Here's how the part is built. I have some questions about the finished solid (model axes, mm). Face numbers are marked on the shaded views. A direction names the side the tool comes from. Give positions to 0.01 mm unless a question says otherwise; leave off trailing zeros. Write each loop counter-clockwise with the first axis right and the second up, starting at its lowest first coordinate (ties: lowest second). Pieces come first, ordered by that corner, then holes. Notation, with made-up numbers: (6, 82) -> (35, 82) arc R17 ccw to (35, 97) -> close; hole circle Ø4 at (-7.5, -19). An arc over 180 degrees is marked (long way). Use one line per item in the form item = value.
```python
from build123d import *

# Parameters (mm, degrees)
F0_R      = 38.1
F1_DEPTH  = 3.175
F3_R      = 31.75
F4_DEPTH  = 1.905
F5_R      = 25.4
F6_DEPTH  = 1.27
F7_R      = 19.05
F8_DEPTH  = 0.635
F10_DEPTH = 10.161
F11_R     = 5.08
F15_R     = 2.54
F16_R     = 0.508


# Not quite as in the source:
# - a fillet or chamfer that OpenCascade refuses, or shapes differently, is made with other operations: its cross-section is extruded or revolved along the edge and cut away or added


with BuildPart() as f1:
    # F0 (on Top) → F1 (new body, symmetric)
    with BuildSketch(Plane.XY):
        Circle(F0_R)
    extrude(amount=F1_DEPTH, both=True)

    # F3 (on face) → F4 (join)
    with BuildSketch(Plane.XY.offset(3.175)):
        Circle(F3_R)
    extrude(amount=F4_DEPTH)

    # F5 (on face) → F6 (join)
    with BuildSketch(Plane.XY.offset(5.08)):
        Circle(F5_R)
    extrude(amount=F6_DEPTH)

    # F7 (on face) → F8 (join)
    with BuildSketch(Plane.XY.offset(6.35)):
        Circle(F7_R)
    extrude(amount=F8_DEPTH)

    # F9 (on face) → F10 (cut, through all)
    with BuildSketch(Plane(origin=(0, 0, -3.175), x_dir=(1, 0, 0), z_dir=(0, 0, -1))):
        Polygon((-6.8075360054, 1.8716637263), (-17.0388379885, -5.08), (-4.3994090512, -5.08), (0, -17.78), (4.3994090512, -5.08), (17.0388379885, -5.08), (6.8075360054, 1.8716637263), (10.9985226281, 13.97), (0, 6.4970477871), (-10.9985226281, 13.97), align=None)
    extrude(amount=-F10_DEPTH, mode=Mode.SUBTRACT)

    # F11
    f11_edges = [f1.edges().sort_by_distance(p)[0] for p in [
        (-38.1, 0, 3.175),
    ]]
    fillet(f11_edges, radius=F11_R)

    # F12: fillet of radius 7.62 on 1 edges, made by hand

    # F12_s1 → F12_t2 (revolve, cut)
    with BuildSketch(Plane.XZ):
        with BuildLine():
            ThreePointArc((31.75, 3.175), (29.4039205887, 4.5878573218), (26.7098437524, 5.08))
            Line((26.7098437524, 5.08), (31.75, 5.08))
            Line((31.75, 5.08), (31.75, 3.175))
        make_face()
    revolve(axis=Axis((0, 0, 5.08), (0, 0, 1)), mode=Mode.SUBTRACT)

    # F13: fillet of radius 7.62 on 1 edges, made by hand

    # F13_s1 → F13_t2 (revolve, cut)
    with BuildSketch(Plane.XZ):
        with BuildLine():
            ThreePointArc((25.4, 5.08), (23.3875910419, 6.0255945611), (21.1878865162, 6.35))
            Line((21.1878865162, 6.35), (25.4, 6.35))
            Line((25.4, 6.35), (25.4, 5.08))
        make_face()
    revolve(axis=Axis((0, 0, 6.35), (0, 0, 1)), mode=Mode.SUBTRACT)

    # F14: fillet of radius 7.62 on 1 edges, made by hand

    # F14_s1 → F14_t2 (revolve, cut)
    with BuildSketch(Plane.XZ):
        with BuildLine():
            ThreePointArc((16.0046469827, 6.985), (17.5600729694, 6.824560979), (19.05, 6.35))
            Line((19.05, 6.35), (19.05, 6.985))
            Line((19.05, 6.985), (16.0046469827, 6.985))
        make_face()
    revolve(axis=Axis((0, 0, 6.985), (0, 0, 1)), mode=Mode.SUBTRACT)

    # F15
    f15_edges = [f1.edges().sort_by_distance(p)[0] for p in [
        (4.399409, 5.08, 1.905),
        (-4.399409, 5.08, 1.905),
        (-6.807536, -1.871664, 1.905),
        (0, -6.497048, 1.905),
        (6.807536, -1.871664, 1.905),
    ]]
    fillet(f15_edges, radius=F15_R)

    # F16
    f16_edges = [f1.edges().sort_by_distance(p)[0] for p in [
        (-10.998523, -13.97, 1.800149),
        (-17.038838, 5.08, 1.800149),
        (0, 17.78, 1.800149),
        (17.038838, 5.08, 1.800149),
        (10.998523, -13.97, 1.800149),
    ]]
    fillet(f16_edges, radius=F16_R)


solid = f1.part
```
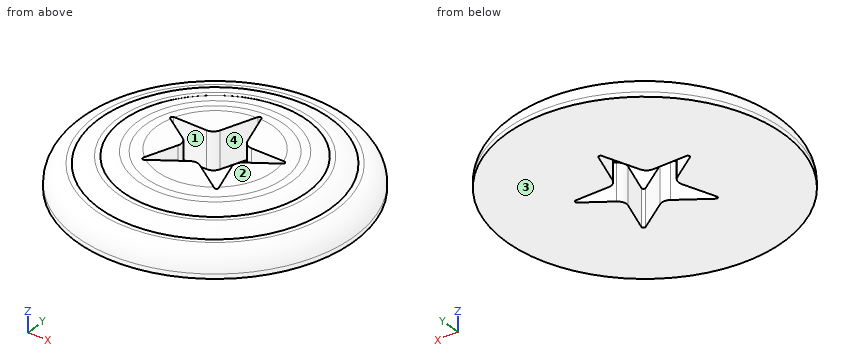
Q1. If I drill on line 1 along X through (y, z) = (-10, 1.5); line 2 along Y through (x, z) = (6, 3.5); line 3 along X through (y, z) = (12.5, -1), over which ranges is the centre line in solid material (lowest first)? Write a range as from..to.
Result set:
line_1 = -35.4..-9.62, -5.16..5.16, 9.62..35.4
line_2 = -30.78..-10.57, 5.09..30.78
line_3 = -35.91..-1.83, 1.83..35.91
Q2. If we mould it in two halves opening along X, with no side actions, what happens to the marked faces 3 and 4? For each: +X half, -X half, draft (parallel to the pull), parting line (faces both ways), or undercut.
Result set:
face_3 = draft
face_4 = undercut
Q3. Will these pins go through, and if not, where does the flat tip stop? pin 1 Ø6 at (y, z) = (-29.5, -2) entering from +X; pin 2 Ø6 at (y, z) = (-15, 4) entering from +X; pin 3 Ø1.5 at (x, y) = (0, -20.5) entering from +Z.
Result set:
pin_1 = 27.37
pin_2 = 34.33
pin_3 = 6.35
Q4. I want a section at A-A, the plane z = -0.5. Write out the boundary of the cut face in (x, y), and give its area (3 significant figures).
Result set:
outline = circle Ø75.8 at (0, 0); hole (-15.67, 4.15) -> (-8.42, -0.78) arc R2.54 cw to (-7.44, -3.71) -> (-10.5, -12.52) arc R0.51 ccw to (-9.73, -13.11) -> (-1.43, -7.47) arc R2.54 cw to (1.43, -7.47) -> (9.73, -13.11) arc R0.51 ccw to (10.5, -12.52) -> (7.44, -3.71) arc R2.54 cw to (8.42, -0.78) -> (15.67, 4.15) arc R0.51 ccw to (15.39, 5.08) -> (6.21, 5.08) arc R2.54 cw to (3.81, 6.79) -> (0.48, 16.39) arc R0.51 ccw to (-0.48, 16.39) -> (-3.81, 6.79) arc R2.54 cw to (-6.21, 5.08) -> (-15.39, 5.08) arc R0.51 ccw to start
area = 4,160 mm2
Q5. Which directions (+Z, -Z, +X, -X, +Y, -Y) give clear straight access to the entire face, cutting with the end or side of a thin tool? Please do the marked faces 1 and 2.
Result set:
face_1 = +Z, -Z
face_2 = +Z, +X, -X, +Y, -Y
